from build123d import *

# Parameters (mm, degrees)
SKETCH_2_W               = 200
SKETCH_2_H               = 50
EXTRUDE_1_DEPTH          = 8
SKETCH_5_W               = 8
SKETCH_5_H               = 20
EXTRUDE_6_DEPTH          = 33
SKETCH_7_W               = 216
SKETCH_7_H               = 20
EXTRUDE_7_DEPTH          = 10
SKETCH_8_W               = 140
SKETCH_8_H               = 8
EXTRUDE_8_DEPTH          = 8
SKETCH_9_W               = 140
SKETCH_9_H               = 10
EXTRUDE_9_DEPTH          = 24
SKETCH_10_W              = 20
SKETCH_10_H              = 8
EXTRUDE_10_DEPTH         = 30
FILLET_1_R               = 2
SKETCH_11_W              = 40
SKETCH_11_H              = 20
EXTRUDE_11_DEPTH         = 25
CUT_EXTRUDE_1_DEPTH      = 148.676305673
CUT_EXTRUDE_1_DEPTH_BACK = 148.676305673
SKETCH_12_W              = 28
SKETCH_12_H              = 16
SKETCH_13_W              = 20
SKETCH_13_H              = 33
EXTRUDE_12_DEPTH         = 25
SKETCH_14_W              = 20
SKETCH_14_H              = 33
EXTRUDE_13_DEPTH         = 25
CUT_EXTRUDE_2_DEPTH      = 170.429357345
CUT_EXTRUDE_2_DEPTH_BACK = 170.429357345
SKETCH_15_W              = 17
SKETCH_15_H              = 20
FILLET_2_R               = 1


with BuildPart() as part:
    # 스케치2 → 보스-돌출1 (new body)
    with BuildSketch(Plane(origin=(0, 0, 0), x_dir=(1, 0, 0), z_dir=(0, 1, 0))):
        with Locations((-17.46031746, 73.968253968)):
            Rectangle(SKETCH_2_W, SKETCH_2_H)
    extrude(amount=EXTRUDE_1_DEPTH)

    # 스케치5 → 보스-돌출6 (add)
    with BuildSketch(Plane.XZ.offset(-33)):
        with Locations((-121.46031746, -88.968253968)):
            Rectangle(SKETCH_5_W, SKETCH_5_H)
        with Locations((86.53968254, -88.968253968)):
            Rectangle(SKETCH_5_W, SKETCH_5_H)
    extrude(amount=EXTRUDE_6_DEPTH)

    # 스케치7 → 보스-돌출7 (add)
    with BuildSketch(Plane(origin=(0, 33, 0), x_dir=(1, 0, 0), z_dir=(0, 1, 0))):
        with Locations((-17.46031746, 88.968253968)):
            Rectangle(SKETCH_7_W, SKETCH_7_H)
    extrude(amount=EXTRUDE_7_DEPTH)

    # 스케치8 → 보스-돌출8 (add)
    with BuildSketch(Plane(origin=(0, 8, 0), x_dir=(1, 0, 0), z_dir=(0, 1, 0))):
        with Locations((-17.46031746, 44.968253968)):
            Rectangle(SKETCH_8_W, SKETCH_8_H)
    extrude(amount=-EXTRUDE_8_DEPTH)

    # 스케치9 → 보스-돌출9 (add)
    with BuildSketch(Plane(origin=(0, 8, 0), x_dir=(1, 0, 0), z_dir=(0, 1, 0))):
        with Locations((-17.46031746, 103.968253968)):
            Rectangle(SKETCH_9_W, SKETCH_9_H)
    extrude(amount=-EXTRUDE_9_DEPTH)

    # 스케치10 → 보스-돌출10 (add)
    with BuildSketch(Plane.XY.offset(-98.968253968)):
        with Locations((-77.46031746, -12)):
            Rectangle(SKETCH_10_W, SKETCH_10_H)
        with Locations((42.53968254, -12)):
            Rectangle(SKETCH_10_W, SKETCH_10_H)
    extrude(amount=EXTRUDE_10_DEPTH)

    # 필렛1
    fillet_1_edges = [part.edges().sort_by_distance(p)[0] for p in [
        (-87.46031746, 4, -40.968253968),
        (52.53968254, 4, -40.968253968),
        (-17.46031746, 8, -40.968253968),
    ]]
    fillet(fillet_1_edges, radius=FILLET_1_R)

    # 스케치11 → 보스-돌출11 (add)
    with BuildSketch(Plane(origin=(0, 43, 0), x_dir=(1, 0, 0), z_dir=(0, 1, 0))):
        with Locations((-105.46031746, 88.968253968)):
            Rectangle(SKETCH_11_W, SKETCH_11_H)
        with Locations((70.53968254, 88.968253968)):
            Rectangle(SKETCH_11_W, SKETCH_11_H)
    extrude(amount=EXTRUDE_11_DEPTH)

    # 스케치12 → 컷-돌출1 (cut, two sides: drawn at the far end of the back side and taken through both)
    with BuildSketch(Plane.XY.offset(-78.968253968).offset(-CUT_EXTRUDE_1_DEPTH_BACK)):
        with Locations((-105.46031746, 51)):
            Rectangle(SKETCH_12_W, SKETCH_12_H)
        with Locations((70.53968254, 51)):
            Rectangle(SKETCH_12_W, SKETCH_12_H)
    extrude(amount=CUT_EXTRUDE_1_DEPTH + CUT_EXTRUDE_1_DEPTH_BACK, mode=Mode.SUBTRACT)

    # 스케치13 → 보스-돌출12 (add)
    with BuildSketch(Plane(origin=(90.53968254, 0, 0), x_dir=(0, 0, -1), z_dir=(1, 0, 0))):
        with Locations((88.968253968, 16.5)):
            Rectangle(SKETCH_13_W, SKETCH_13_H)
    extrude(amount=EXTRUDE_12_DEPTH)

    # 스케치14 → 보스-돌출13 (add)
    with BuildSketch(Plane.ZY.offset(125.46031746)):
        with Locations((-88.968253968, 16.5)):
            Rectangle(SKETCH_14_W, SKETCH_14_H)
    extrude(amount=EXTRUDE_13_DEPTH)

    # 스케치15 → 컷-돌출2 (cut, two sides: drawn at the far end of the back side and taken through both)
    with BuildSketch(Plane.XY.offset(-78.968253968).offset(-CUT_EXTRUDE_2_DEPTH_BACK)):
        with Locations((-133.96031746, 16.5)):
            Rectangle(SKETCH_15_W, SKETCH_15_H)
        with Locations((99.03968254, 16.5)):
            Rectangle(SKETCH_15_W, SKETCH_15_H)
    extrude(amount=CUT_EXTRUDE_2_DEPTH + CUT_EXTRUDE_2_DEPTH_BACK, mode=Mode.SUBTRACT)

    # 필렛2
    fillet_2_edges = [part.edges().sort_by_distance(p)[0] for p in [
        (-85.46031746, 43, -88.968253968),
        (-125.46031746, 68, -88.968253968),
        (-85.46031746, 68, -88.968253968),
        (50.53968254, 43, -88.968253968),
        (50.53968254, 68, -88.968253968),
        (90.53968254, 68, -88.968253968),
        (-91.46031746, 59, -88.968253968),
        (-91.46031746, 43, -88.968253968),
        (-119.46031746, 43, -88.968253968),
        (-119.46031746, 59, -88.968253968),
        (84.53968254, 59, -88.968253968),
        (84.53968254, 43, -88.968253968),
        (56.53968254, 43, -88.968253968),
        (56.53968254, 59, -88.968253968),
        (90.53968254, 33, -88.968253968),
        (115.53968254, 0, -88.968253968),
        (115.53968254, 33, -88.968253968),
        (-125.46031746, 33, -88.968253968),
        (-150.46031746, 0, -88.968253968),
        (-150.46031746, 33, -88.968253968),
        (-142.46031746, 6.5, -88.968253968),
        (-142.46031746, 26.5, -88.968253968),
        (-125.46031746, 26.5, -88.968253968),
        (-125.46031746, 6.5, -88.968253968),
        (90.53968254, 6.5, -88.968253968),
        (90.53968254, 26.5, -88.968253968),
        (107.53968254, 26.5, -88.968253968),
        (107.53968254, 6.5, -88.968253968),
    ]]
    fillet(fillet_2_edges, radius=FILLET_2_R)


solid = part.part
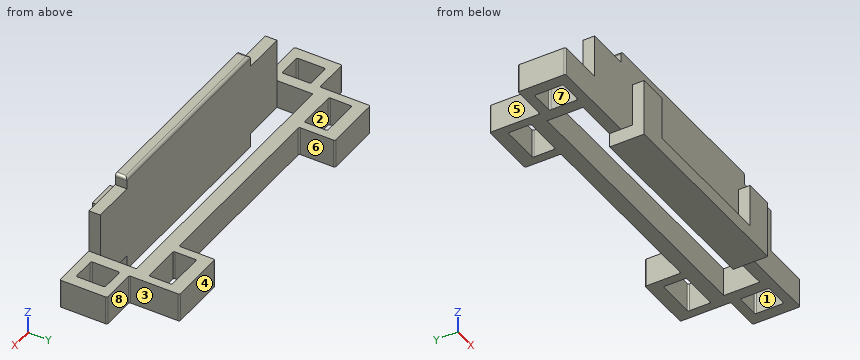
Input: part model. Units: mm. Frame: model coordinates. Face numbers are marked on the shaded views. A direction names the side the tool comes from. Coordinates: 2 decimals unless noted, no trailing zeros. Order: outer loops, then holes, each group sorted by start corner. A loop starts at its lowest first (then second) coordinate and runs counter-clockwise, first axis right, second up. Notation, with made-up numbers: M 4,-2 L 11,-2 A24 cw 11,23 Z; hole C 5,-25.5 d6. An arc over 180 degrees is marked long. One line per question, with ' | ' between items.
Item 1: Pin query (flat end, axial travel): pin 1 (12 mm diameter, centred on y = -2.5, z = -69, fed in from +X); pin 2 (9 mm diameter, centred on x = 63.5, y = 5, fed in from +Z); pin 3 (9 mm diameter, centred on y = 3, z = -65, fed in from -X); pin 4 (16.5 mm diameter, centred on x = -131, z = -88.5, fed in from +Y). Return the tip coordinate at first contact, or that it passes through.
Geometry results:
pin 1: stops at x = 82.54 | pin 2: stops at z = -48.97 | pin 3: stops at x = -117.46 | pin 4: stops at y = 68
Item 2: Section C-C (x = -18.5). Output: boundary loops of the cut face in (y, z).
Geometry results:
outline: M -16,-108.97 L 8,-108.97 L 8,-42.97 A2 ccw 6,-40.97 L 0,-40.97 L 0,-98.97 L -16,-98.97 Z; M 33,-98.97 L 43,-98.97 L 43,-78.97 L 33,-78.97 Z
Item 3: Section A-A (y = 22.5). Output: boundary loops of the cut face in (x, z), then the cut area to 3 significant figures.
Geometry results:
outline: M -150.46,-98.97 L -142.46,-98.97 L -142.46,-78.97 L -150.46,-78.97 Z; M -125.46,-98.97 L -117.46,-98.97 L -117.46,-78.97 L -125.46,-78.97 Z; M 82.54,-98.97 L 90.54,-98.97 L 90.54,-78.97 L 82.54,-78.97 Z; M 107.54,-98.97 L 115.54,-98.97 L 115.54,-78.97 L 107.54,-78.97 Z | area: 640 mm^2
Item 4: Section B-B (z = -74.5). Output: boundary loops of the cut face in (x, y), then the cut area to 3 significant figures.
Geometry results:
outline: M -117.46,0 L 82.54,0 L 82.54,8 L -117.46,8 Z; M -87.46,-16 L -67.46,-16 L -67.46,-8 L -87.46,-8 Z; M 32.54,-16 L 52.54,-16 L 52.54,-8 L 32.54,-8 Z | area: 1,920 mm^2
Item 5: Ray query, line 1 along Y through (x, z) = (49, -97); line 2 along X through (y, z) = (8.5, -83.5); line 3 along Y through (x, z) = (11, -87). Return the intervals inside material, ascending.
Geometry results:
line 1: y = -16 to -8, 0 to 8, 33 to 43 | line 2: x = -150.46 to -142.46, -125.46 to -117.46, 82.54 to 90.54, 107.54 to 115.54 | line 3: y = 0 to 8, 33 to 43
Item 6: Reachability of the marked faces 5, 6, 7 and 8 from +Z, -Z, +X, -X, +Y, -Y: full face, straight path, thin tool, end or side. Return the list, or none.
Geometry results:
face 5: +Z, -Z, -X, +Y | face 6: +Z, -Z, +Y | face 7: +Z, -Z | face 8: +Z, -Z, +X, +Y
Item 7: Draft query along Y for the marked faces 1, 2, 3 and 4. Return one class per face: released by +Y, released by -Y, zero draft, split by the parting line, or undercut.
Geometry results:
face 1: undercut | face 2: undercut | face 3: zero draft | face 4: released by +Y
Item 8: Section D-D (z = -91). Give the number of separate pieces and of enclosed holes in the cut face, then the cut area to 3 significant figures.
Geometry results:
separate pieces: 3 | enclosed holes: 5 | area: 6,680 mm^2
